from build123d import *

# Parameters (mm, degrees)
SKETCH1_W           = 119.38
SKETCH1_H           = 119.38
BOSS_EXTRUDE1_DEPTH = 4.7625
CUT_EXTRUDE1_REACH  = 131.937
SKETCH2_R           = 2.286
SKETCH2_R_2         = 1.27
SKETCH2_R_3         = 55.42912263
CUT_EXTRUDE2_REACH  = 131.937
SKETCH4_W           = 14.986
SKETCH4_H           = 17.78
FILLET2_R           = 2.54
FILLET3_R           = 2.54


with BuildPart() as part:
    # Sketch1 → Boss-Extrude1 (new body)
    with BuildSketch(Plane.XY):
        with Locations((-31.19657191, 33.049217791)):
            Rectangle(SKETCH1_W, SKETCH1_H)
    extrude(amount=BOSS_EXTRUDE1_DEPTH)

    # Sketch2 → Cut-Extrude1 (cut, up to next)
    with BuildSketch(Plane(origin=(0, 0, 0), x_dir=(-1, 0, 0), z_dir=(0, 0, -1)), mode=Mode.PRIVATE) as cut_extrude1_sk1:
        with Locations((-21.25442809, 85.500217791)):
            Circle(SKETCH2_R)
    cut_extrude1_tool1 = extrude(cut_extrude1_sk1.sketch, amount=-CUT_EXTRUDE1_REACH, mode=Mode.PRIVATE) & part.part
    # Sketch2 → Cut-Extrude1 (cut, up to next)
    with BuildSketch(Plane(origin=(0, 0, 0), x_dir=(-1, 0, 0), z_dir=(0, 0, -1)), mode=Mode.PRIVATE) as cut_extrude1_sk2:
        with Locations((83.64757191, 85.500217791)):
            Circle(SKETCH2_R)
    cut_extrude1_tool2 = extrude(cut_extrude1_sk2.sketch, amount=-CUT_EXTRUDE1_REACH, mode=Mode.PRIVATE) & part.part
    # Sketch2 → Cut-Extrude1 (cut, up to next)
    with BuildSketch(Plane(origin=(0, 0, 0), x_dir=(-1, 0, 0), z_dir=(0, 0, -1)), mode=Mode.PRIVATE) as cut_extrude1_sk3:
        with Locations(Location((72.09057191, -12.988282209, 0), (0, 0, 180))):
            Circle(SKETCH2_R_2)
    cut_extrude1_tool3 = extrude(cut_extrude1_sk3.sketch, amount=-CUT_EXTRUDE1_REACH, mode=Mode.PRIVATE) & part.part
    # Sketch2 → Cut-Extrude1 (cut, up to next)
    with BuildSketch(Plane(origin=(0, 0, 0), x_dir=(-1, 0, 0), z_dir=(0, 0, -1)), mode=Mode.PRIVATE) as cut_extrude1_sk4:
        with Locations((31.19657191, 33.049217791)):
            Circle(SKETCH2_R_3)
    cut_extrude1_tool4 = extrude(cut_extrude1_sk4.sketch, amount=-CUT_EXTRUDE1_REACH, mode=Mode.PRIVATE) & part.part
    # Sketch2 → Cut-Extrude1 (cut, up to next)
    with BuildSketch(Plane(origin=(0, 0, 0), x_dir=(-1, 0, 0), z_dir=(0, 0, -1)), mode=Mode.PRIVATE) as cut_extrude1_sk5:
        with Locations((-13.44392809, 77.689717791)):
            Circle(SKETCH2_R_2)
    cut_extrude1_tool5 = extrude(cut_extrude1_sk5.sketch, amount=-CUT_EXTRUDE1_REACH, mode=Mode.PRIVATE) & part.part
    # Sketch2 → Cut-Extrude1 (cut, up to next)
    with BuildSketch(Plane(origin=(0, 0, 0), x_dir=(-1, 0, 0), z_dir=(0, 0, -1)), mode=Mode.PRIVATE) as cut_extrude1_sk6:
        with Locations(Location((75.83707191, 77.689717791, 0), (0, 0, 180))):
            Circle(SKETCH2_R_2)
    cut_extrude1_tool6 = extrude(cut_extrude1_sk6.sketch, amount=-CUT_EXTRUDE1_REACH, mode=Mode.PRIVATE) & part.part
    # Sketch2 → Cut-Extrude1 (cut, up to next)
    with BuildSketch(Plane(origin=(0, 0, 0), x_dir=(-1, 0, 0), z_dir=(0, 0, -1)), mode=Mode.PRIVATE) as cut_extrude1_sk7:
        with Locations((-9.69742809, -12.988282209)):
            Circle(SKETCH2_R_2)
    cut_extrude1_tool7 = extrude(cut_extrude1_sk7.sketch, amount=-CUT_EXTRUDE1_REACH, mode=Mode.PRIVATE) & part.part
    add(cut_extrude1_tool1.solids().sort_by_distance((21.254428, 85.500218, 0))[0], mode=Mode.SUBTRACT)
    add(cut_extrude1_tool2.solids().sort_by_distance((-83.647572, 85.500218, 0))[0], mode=Mode.SUBTRACT)
    add(cut_extrude1_tool3.solids().sort_by_distance((-72.090572, -12.988282, 0))[0], mode=Mode.SUBTRACT)
    add(cut_extrude1_tool4.solids().sort_by_distance((-31.196572, 33.049218, 0))[0], mode=Mode.SUBTRACT)
    add(cut_extrude1_tool5.solids().sort_by_distance((13.443928, 77.689718, 0))[0], mode=Mode.SUBTRACT)
    add(cut_extrude1_tool6.solids().sort_by_distance((-75.837072, 77.689718, 0))[0], mode=Mode.SUBTRACT)
    add(cut_extrude1_tool7.solids().sort_by_distance((9.697428, -12.988282, 0))[0], mode=Mode.SUBTRACT)

    # Sketch4 → Cut-Extrude2 (cut, up to next)
    with BuildSketch(Plane(origin=(0, 0, 0), x_dir=(-1, 0, 0), z_dir=(0, 0, -1)), mode=Mode.PRIVATE) as cut_extrude2_sk1:
        with Locations((-21.00042809, -17.750782209)):
            Rectangle(SKETCH4_W, SKETCH4_H)
    cut_extrude2_tool1 = extrude(cut_extrude2_sk1.sketch, amount=-CUT_EXTRUDE2_REACH, mode=Mode.PRIVATE) & part.part
    # Sketch4 → Cut-Extrude2 (cut, up to next)
    with BuildSketch(Plane(origin=(0, 0, 0), x_dir=(-1, 0, 0), z_dir=(0, 0, -1)), mode=Mode.PRIVATE) as cut_extrude2_sk2:
        with Locations((83.39357191, -17.750782209)):
            Rectangle(SKETCH4_W, SKETCH4_H)
    cut_extrude2_tool2 = extrude(cut_extrude2_sk2.sketch, amount=-CUT_EXTRUDE2_REACH, mode=Mode.PRIVATE) & part.part
    add(cut_extrude2_tool1.solids().sort_by_distance((21.000428, -17.750782, 0))[0], mode=Mode.SUBTRACT)
    add(cut_extrude2_tool2.solids().sort_by_distance((-83.393572, -17.750782, 0))[0], mode=Mode.SUBTRACT)

    # Fillet2
    fillet2_edges = [part.edges().sort_by_distance(p)[0] for p in [
        (-90.88657191, 92.739217791, 2.38125),
        (28.49342809, 92.739217791, 2.38125),
    ]]
    fillet(fillet2_edges, radius=FILLET2_R)

    # Fillet3
    fillet3_edges = [part.edges().sort_by_distance(p)[0] for p in [
        (28.49342809, -8.860782209, 2.38125),
        (13.50742809, -26.640782209, 2.38125),
        (-75.90057191, -26.640782209, 2.38125),
        (-90.88657191, -8.860782209, 2.38125),
    ]]
    fillet(fillet3_edges, radius=FILLET3_R)


solid = part.part
Can you work these out from the model? Positions are in its coordinate system, mm. A direction names the side the tool comes from. Coordinates: 2 decimals unless noted, no trailing zeros. Loops run counter-clockwise (first coordinate to the right, second up) from the corner with the lowest first, then second, coordinate; pieces in that order, holes last. Notation, with made-up numbers: M 39.5,20.25 L 81.5,20.25 A17 ccw 81.5,31.25 Z; hole C -8,60 d2. An arc over 180 degrees is marked long. Return JSON: item names as keys, results as strings. Group by question number.
Item 1: I'm going to push flat-ended pins straight in: pin 1 Ø1.4 at (x, z) = (-83.5, 3.5) entering from -Y; pin 2 Ø2.5 at (y, z) = (-18.5, 1.5) entering from -X. Where does each tip first touch, or does it pass through?
Item 2: On a 3-axis mill with a long thin cutter (end or side, diameter ignored), from which of +Z, -Z, +X, -X, +Y, -Y can I reach the whole of each face in a straight line? I mean faces 1 (the flat face through (-82, -8.861, 2)), 2 (the flat face through (13.507, -17, 2)), 3 (the cylindrical face through (13.72, 76.45, 2.35)). Say none if no direction works.
Item 3: Thinking about a two-plate mould opening in X: for faces 4 (the flat face through (28.493, 41, 2)), 5 (the cylindrical face through (8.524, -13.475, 2.348)), 6 (the flat face through (20, -8.861, 2)), which applies, released by +X, released by -X, zero draft, split by the parting line, or undercut?
Item 4: Imagine slicing it at C-C (z = 2.35). Please give me the cut outline in (x, y), and give its area (3 significant figures).
Item 5: If I drill on L1, parallel to Y at x = -76.5, z = 2.4; L2, parallel to X at y = 33, z = 3.7; L3, parallel to Y at x = -16.5, z = 3.2, over which ranges is the centre line in solid material (lowest first)? Write a range as from..to.
Item 6: Imagine slicing it at A-A (y = 59.5). Please give me the cut outline in (x, z), and give its area (3 significant figures).
Item 7: Imagine slicing it at B-B (x = -38). Please give me the cut outline in (y, z).
Verdict:
{
 "1": {"pin 1": "stops at y = -8.86", "pin 2": "stops at x = -75.9"},
 "2": {"face 1": "+Z, -Z, -X, -Y", "face 2": "+Z, -Z, +X, -Y", "face 3": "+Z, -Z"},
 "3": {"face 4": "released by +X", "face 5": "undercut", "face 6": "zero draft"},
 "4": {"outline": "M -90.89,-6.32 A2.54 ccw -88.35,-8.86 L -75.9,-8.86 L -75.9,-24.1 A2.54 ccw -73.36,-26.64 L 10.97,-26.64 A2.54 ccw 13.51,-24.1 L 13.51,-8.86 L 25.95,-8.86 A2.54 ccw 28.49,-6.32 L 28.49,90.2 A2.54 ccw 25.95,92.74 L -88.35,92.74 A2.54 ccw -90.89,90.2 Z; hole C -31.2,33.05 d110.86; hole C -83.65,85.5 d4.57; hole C -75.84,77.69 d2.54; hole C -72.09,-12.99 d2.54; hole C 9.7,-12.99 d2.54; hole C 13.44,77.69 d2.54; hole C 21.25,85.5 d4.57", "area": "4,010 mm^2"},
 "5": {"L1": "y = -8.86..1.11, 64.99..76.61, 78.77..92.74", "L2": "x = -90.89..-86.63, 24.23..28.49", "L3": "y = -26.64..-20.4, 86.49..92.74"},
 "6": {"outline": "M -90.89,0 L -79.91,0 L -79.91,4.76 L -90.89,4.76 Z; M 17.51,0 L 28.49,0 L 28.49,4.76 L 17.51,4.76 Z", "area": "105 mm^2"},
 "7": {"outline": "M -26.64,0 L -21.96,0 L -21.96,4.76 L -26.64,4.76 Z; M 88.06,0 L 92.74,0 L 92.74,4.76 L 88.06,4.76 Z"}
}
